from build123d import *

# Parameters (mm, degrees)
SKETCH1_W                 = 12.7
SKETCH1_H                 = 6.35
BOSS_EXTRUDE1_DEPTH       = 50.8
SKETCH2_W                 = 50.8
SKETCH2_H                 = 19.05
BOSS_EXTRUDE2_DEPTH       = 7.35076
M3X0_5_TAPPED_HOLE1_D     = 2.5
M3X0_5_TAPPED_HOLE1_DEPTH = 6.35
M3X0_5_TAPPED_HOLE1_TIP   = 0.751075774
M3X0_5_TAPPED_HOLE2_D     = 2.5
M4_CLEARANCE_HOLE1_D      = 4.5


with BuildPart() as part:
    # Sketch1 → Boss-Extrude1 (new body)
    with BuildSketch(Plane(origin=(0, 0, 0), x_dir=(0, 0, -1), z_dir=(1, 0, 0))):
        Polygon((19.177, 6.35), (19.177, 31.877), (0, 31.877), (0, 25.527), (12.827, 25.527), (12.827, 0), (19.177, 0), align=None)
        with Locations((25.527, 3.175)):
            Rectangle(SKETCH1_W, SKETCH1_H)
        Polygon((0, 25.527), (0, 31.877), (-19.177, 31.877), (-19.177, 6.35), (-19.177, 0), (-12.827, 0), (-12.827, 25.527), align=None)
        with Locations((-25.527, 3.175)):
            Rectangle(SKETCH1_W, SKETCH1_H)
    extrude(amount=BOSS_EXTRUDE1_DEPTH)

    # Sketch2 → Boss-Extrude2 (add)
    with BuildSketch(Plane(origin=(0, 31.877, 0), x_dir=(1, 0, 0), z_dir=(0, 1, 0))):
        with Locations((25.4, 0)):
            Rectangle(SKETCH2_W, SKETCH2_H)
    extrude(amount=BOSS_EXTRUDE2_DEPTH)

    # M3x0.5 Tapped Hole1
    with Locations(Plane(origin=(0, 39.22776, 0), x_dir=(1, 0, 0), z_dir=(0, 1, 0))):
        with Locations((25.4, -6.985), (25.4, 6.985)):
            Hole(M3X0_5_TAPPED_HOLE1_D / 2, depth=M3X0_5_TAPPED_HOLE1_DEPTH)
            with Locations((0, 0, -(M3X0_5_TAPPED_HOLE1_DEPTH + M3X0_5_TAPPED_HOLE1_TIP / 2))):  # 118° drill point
                Cone(0, M3X0_5_TAPPED_HOLE1_D / 2, M3X0_5_TAPPED_HOLE1_TIP, mode=Mode.SUBTRACT)

    # M3x0.5 Tapped Hole2 (through all)
    with Locations(Plane(origin=(0, 31.877, 0), x_dir=(1, 0, 0), z_dir=(0, 1, 0))):
        with Locations((38.1, 14.351), (12.7, 14.351)):
            m3x0_5_tapped_hole2 = Hole(M3X0_5_TAPPED_HOLE2_D / 2)

    # Mirror1: M3x0.5 Tapped Hole2 across plane
    add(m3x0_5_tapped_hole2.mirror(Plane.XY), mode=Mode.SUBTRACT)

    # M4 Clearance Hole1 (through all)
    with Locations(Plane(origin=(0, 6.35, 0), x_dir=(1, 0, 0), z_dir=(0, 1, 0))):
        with Locations((41.275, 25.527), (9.525, 25.527)):
            m4_clearance_hole1 = Hole(M4_CLEARANCE_HOLE1_D / 2)

    # Mirror2: M4 Clearance Hole1 across plane
    add(m4_clearance_hole1.mirror(Plane.XY), mode=Mode.SUBTRACT)


solid = part.part
Can you work these out from the model? Positions are in its coordinate system, mm. A direction names the side the tool comes from. Coordinates: 2 decimals unless noted, no trailing zeros. Write each loop counter-clockwise with the first axis right and the second up, starting at its lowest first coordinate (ties: lowest second). Pieces come first, ordered by that corner, then holes. Notation, with made-up numbers: (33, 33) - (57, 33) arc R34 cw to (57, 67) - close; hole circle Ø8 at (21.25, 85). An arc over 180 degrees is marked (long way). Return JSON: item names as keys, results as strings. Group by question number.
Item 1: If we section it at B-B (x = 30.5): Write out the boundary of the cut face in (y, z) (3 decimals).
Item 2: If we section it at D-D (z = 1.5): Write out the boundary of the cut face in (x, y), then the cut area to 3 significant figures.
Item 3: If we section it at A-A (x = 12.7): Write out the boundary of the cut face in (y, z) (3 decimals), then the cut area to 3 significant figures.
Item 4: If we section it at C-C (y = 35.5): Write out the boundary of the cut face in (x, z) (3 decimals).
Item 5: I'm going to push flat-ended pins straight in: pin 1 Ø12 at (x, y) = (5.5, 19.5) entering from +Z; pin 2 Ø14 at (x, z) = (35.5, 28) entering from +Y; pin 3 Ø2 at (x, y) = (25.5, 36) entering from -Z (3 decimals); pin 4 Ø3.5 at (x, z) = (9.525, -25.527) entering from +Y. Where does each tip first touch, or does it pass through?
Item 6: We'd pull the mould along X, two halves only. Please class faces 5 (the face through (25, 31.877, -14)), 6 (the face through (43.06, 3.13, -24.16)), 7 (the face through (50.8, 27, 5)): pulls with the +X half, pulls with the -X half, needs draft (parallel to the pull), parting line crosses it, or undercut.
Item 7: Please list where these lines run through material, in increasing order: probe 1 along Z at (x, y) = (38, 11) (3 decimals); probe 2 along Z at (x, y) = (25.4, 37.75) (3 decimals); probe 3 along Z at (x, y) = (3, 2).
Item 8: Which directions (+Z, -Z, +X, -X, +Y, -Y) give clear straight access to the entire face, cutting with the end or side of a thin tool? Please do faces 1 (the face through (25, 6.35, -25)), 2 (the face through (25, 31.877, 14)), 3 (the face through (25, 13, -12.827)), 4 (the face through (26.65, 36.01, -7.04)).
Return value:
{
 "1": {"outline": "(0, -31.877) - (6.35, -31.877) - (6.35, -19.177) - (31.877, -19.177) - (31.877, -9.525) - (39.228, -9.525) - (39.228, 9.525) - (31.877, 9.525) - (31.877, 19.177) - (6.35, 19.177) - (6.35, 31.877) - (0, 31.877) - (0, 12.827) - (25.527, 12.827) - (25.527, -12.827) - (0, -12.827) - close"},
 "2": {"outline": "(0, 25.53) - (50.8, 25.53) - (50.8, 39.23) - (0, 39.23) - close", "area": "696 mm^2"},
 "3": {"outline": "(0, -31.877) - (6.35, -31.877) - (6.35, -19.177) - (31.877, -19.177) - (31.877, -15.601) - (0, -15.601) - close; (0, -13.101) - (31.877, -13.101) - (31.877, -9.525) - (39.228, -9.525) - (39.228, 9.525) - (31.877, 9.525) - (31.877, 13.101) - (0, 13.101) - (0, 12.827) - (25.527, 12.827) - (25.527, -12.827) - (0, -12.827) - close; (0, 15.601) - (31.877, 15.601) - (31.877, 19.177) - (6.35, 19.177) - (6.35, 31.877) - (0, 31.877) - close", "area": "710 mm^2"},
 "4": {"outline": "(0, -9.525) - (50.8, -9.525) - (50.8, 9.525) - (0, 9.525) - close; hole circle Ø2.5 at (25.4, -6.985); hole circle Ø2.5 at (25.4, 6.985)"},
 "5": {"pin 1": "stops at z = 19.18", "pin 2": "stops at y = 6.35", "pin 3": "stops at z = -9.525", "pin 4": "passes through"},
 "6": {"face 5": "needs draft", "face 6": "undercut", "face 7": "pulls with the +X half"},
 "7": {"probe 1": "z = -19.177 to -15.597, -13.105 to -12.827, 12.827 to 13.105, 15.597 to 19.177", "probe 2": "z = -9.525 to -8.235, -5.735 to 5.735, 8.235 to 9.525", "probe 3": "z = -31.88 to -12.83, 12.83 to 31.88"},
 "8": {"face 1": "-Z, +X, -X, +Y", "face 2": "+Z, +X, -X, +Y", "face 3": "+X, -X, -Y", "face 4": "+Y"}
}
